Geometry: see drawing. Coordinates: mm, zero at the bounding-box minimum. Round coordinates to 2 decimals unless told otherwise and drop trailing zeros. Order: outer loops, then holes, each group sorted by start corner. A loop starts at its lowest first (then second) coordinate and runs counter-clockwise, first axis right, second up. Notation, with made-up numbers: (-7, 59.25) -> (10, 59.25) arc R25 ccw to (10, 90.25) -> close; hole circle Ø7 at (65.25, 31). An arc over 180 degrees is marked (long way). Use a Markdown table: item, result.
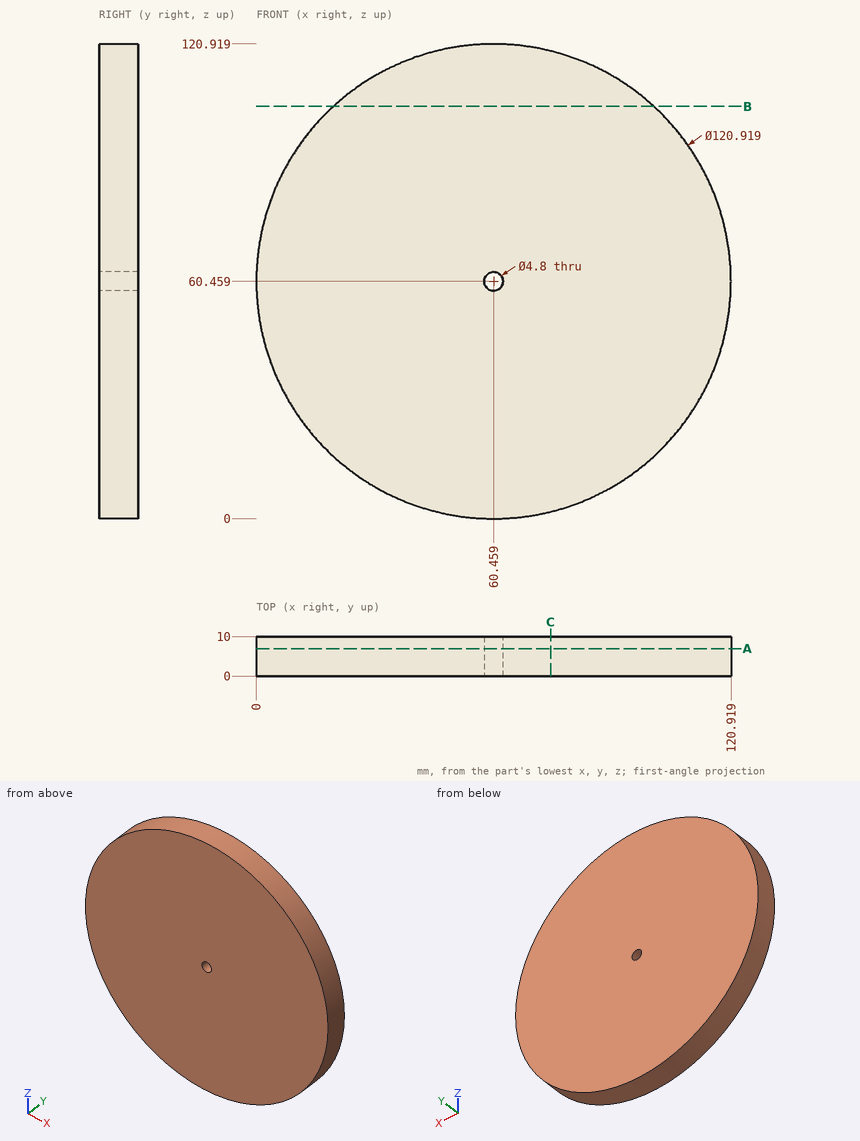
1) Contact query for flat-ended pins moving along their axis: P1, Ø6, axis at x = 34.5, y = 8.5, coming from the -Z side; P2, Ø5, axis at y = 4.5, z = 13.5, coming from the -X side; P3, Ø4, axis at y = 3, z = 102.5, coming from the -X side. Output: stop coordinate, or through.
Answer key:
| item | result |
|---|---|
| P1 | stops at z = 4.53 |
| P2 | stops at x = 19.49 |
| P3 | stops at x = 15.16 |
2) Cut plane B-B on z = 105. Return loops of the section in (x, y) (1 decimal).
Answer key:
| item | result |
|---|---|
| outline | (19.6, 0) -> (101.3, 0) -> (101.3, 10) -> (19.6, 10) -> close |
3) Cut plane C-C on x = 75. Return loops of the section in (y, z) (1 decimal).
Answer key:
| item | result |
|---|---|
| outline | (0, 1.8) -> (10, 1.8) -> (10, 119.1) -> (0, 119.1) -> close |
4) Ray query, probe 1 along X at (y, z) = (2.25, 61); probe 2 along Z at (x, y) = (46, 4) (1 decimal); probe 3 along Z at (x, y) = (101, 2.5) (1 decimal). Return the intervals inside material, ascending.
Answer key:
| item | result |
|---|---|
| probe 1 | x = 0 to 58.12, 62.8 to 120.92 |
| probe 2 | z = 1.8 to 119.2 |
| probe 3 | z = 15.6 to 105.3 |
5) Cut plane A-A on y = 7. Return loops of the section in (x, z), and give its area (3 significant figures).
Answer key:
| item | result |
|---|---|
| outline | circle Ø120.92 at (60.46, 60.46); hole circle Ø4.8 at (60.46, 60.46) |
| area | 11,500 mm^2 |
